```python
from build123d import *

# Parameters (mm, degrees)
ESQUISSE1_W             = 330
ESQUISSE1_H             = 205
BOSS_EXTRU_1_DEPTH      = 30
CHANFREIN1_SIZE         = 30
CHANFREIN1_SIZE2        = 17.320508076
CONG_1_R                = 50
CONG_3_R                = 10
ESQUISSE2_W             = 310
ESQUISSE2_H             = 185
ENL_V_MAT_EXTRU_1_DEPTH = 1
D_GAGEMENT_M42_D        = 4
D_GAGEMENT_M42_DEPTH    = 10
D_GAGEMENT_M42_TIP      = 1.201721238
D_GAGEMENT_M71_D        = 7
D_GAGEMENT_M71_DEPTH    = 5
D_GAGEMENT_M71_TIP      = 2.103012167
ENL_V_MAT_EXTRU_2_DEPTH = 17.320508


with BuildPart() as part:
    # Esquisse1 → Boss.-Extru.1 (new body)
    with BuildSketch(Plane.XY):
        with Locations((165, 102.5)):
            Rectangle(ESQUISSE1_W, ESQUISSE1_H)
    extrude(amount=BOSS_EXTRU_1_DEPTH)

    # Chanfrein1
    chanfrein1_edges = [part.edges().sort_by_distance(p)[0] for p in [
        (165, 205, 0),
        (330, 102.5, 0),
        (165, 0, 0),
        (0, 102.5, 0),
    ]]
    chanfrein1_side = [part.faces().sort_by_distance(p)[0] for p in [
        (165, 102.5, 0),
    ]]
    chamfer(chanfrein1_edges, length=CHANFREIN1_SIZE, length2=CHANFREIN1_SIZE2, reference=chanfrein1_side[0])

    # Congé1
    cong_1_edges = [part.edges().sort_by_distance(p)[0] for p in [
        (315, 15, 8.660254038),
        (15, 15, 8.660254038),
        (315, 190, 8.660254038),
        (15, 190, 8.660254038),
    ]]
    fillet(cong_1_edges, radius=CONG_1_R)

    # Congé3
    cong_3_edges = [part.edges().sort_by_distance(p)[0] for p in [
        (0, 205, 25.524681254),
        (330, 205, 25.524681254),
        (330, 0, 25.524681254),
        (0, 0, 25.524681254),
    ]]
    fillet(cong_3_edges, radius=CONG_3_R)

    # Esquisse2 → Enlèv. mat.-Extru.1 (cut)
    with BuildSketch(Plane.XY.offset(30)):
        with Locations((165, 102.5)):
            Rectangle(ESQUISSE2_W, ESQUISSE2_H)
    extrude(amount=-ENL_V_MAT_EXTRU_1_DEPTH, mode=Mode.SUBTRACT)

    # Dégagement M42
    with Locations(Plane(origin=(0, 0, 0), x_dir=(-1, 0, 0), z_dir=(0, 0, -1))):
        with Locations((-202.5, 65), (-127.5, 140), (-127.5, 65), (-202.5, 140)):
            Hole(D_GAGEMENT_M42_D / 2, depth=D_GAGEMENT_M42_DEPTH)
            with Locations((0, 0, -(D_GAGEMENT_M42_DEPTH + D_GAGEMENT_M42_TIP / 2))):  # 118° drill point
                Cone(0, D_GAGEMENT_M42_D / 2, D_GAGEMENT_M42_TIP, mode=Mode.SUBTRACT)

    # Dégagement M71
    with Locations(Plane(origin=(0, 0, 0), x_dir=(-1, 0, 0), z_dir=(0, 0, -1))):
        with Locations((-215, 152.5), (-115, 152.5), (-165, 42.313793967)):
            Hole(D_GAGEMENT_M71_D / 2, depth=D_GAGEMENT_M71_DEPTH)
            with Locations((0, 0, -(D_GAGEMENT_M71_DEPTH + D_GAGEMENT_M71_TIP / 2))):  # 118° drill point
                Cone(0, D_GAGEMENT_M71_D / 2, D_GAGEMENT_M71_TIP, mode=Mode.SUBTRACT)

    # Esquisse9 → Enlèv. mat.-Extru.2 (cut)
    with BuildSketch(Plane(origin=(0, 0, 0), x_dir=(-1, 0, 0), z_dir=(0, 0, -1))):
        with BuildLine():
            Line((-330, 180), (-297.928932188, 147.928932188))
            ThreePointArc((-297.928932188, 147.928932188), (-295.761204675, 144.6846987), (-295, 140.857864376))
            Line((-295, 140.857864376), (-295, 64.142135624))
            ThreePointArc((-295, 64.142135624), (-295.761204675, 60.3153013), (-297.928932188, 57.071067812))
            Line((-297.928932188, 57.071067812), (-330, 25))
            Line((-330, 25), (-330, 180))
        make_face()
    extrude(amount=-ENL_V_MAT_EXTRU_2_DEPTH, mode=Mode.SUBTRACT)


solid = part.part
```
Geometry: final body of the model. Coordinates: model frame, mm. A direction names the side the tool comes from. Coordinates: 2 decimals unless noted, no trailing zeros. Order: outer loops, then holes, each group sorted by start corner. A loop starts at its lowest first (then second) coordinate and runs counter-clockwise, first axis right, second up. Notation, with made-up numbers: (-27, 63) - (16, 63) arc R19 cw to (16, 79) - close; hole circle Ø8 at (-6.75, 15). An arc over 180 degrees is marked (long way). Return JSON: item names as keys, results as strings. Group by question number.
1. Cut plane B-B (y = 108.5). Output: boundary loops of the cut face in (x, z), plus the area to 3 significant figures.
2. Set-up query: faces 4 (the face through (295.782, 144.735, 8.539)), 5 (the face through (118.233, 151.159, 2.535)), 6 (the face through (163.04, 190.21, 8.78)). Return all of +Z, -Z, +X, -X, +Y, -Y with unobstructed straight access to the full face (end or side cutting, diameter ignored); none if empty.
3. Cut plane A-A (x = 102). Output: boundary loops of the cut face in (y, z).
4. Material intervals for line 1 along Z through (x, y) = (99.5, 168); line 2 along Y through (x, z) = (202, 3); line 3 along Y through (x, z) = (115, 2), sorted ascending. Write a range as [from, to].
5. Pin query (flat end, axial travel): pin 1 (4 mm diameter, centred on x = 156, z = 3, fed in from +Y); pin 2 (1.5 mm diameter, centred on x = 116, z = 12.5, fed in from +Y); pin 3 (6.5 mm diameter, centred on x = 127.5, y = 140, fed in from +Z). Return the tip coordinate at first contact, or that it passes through.
6. Pull-direction query (X, two-part tool) for faces 1 (the face through (310, 45, 10)), 2 (the face through (163, 104, 29)), 3 (the face through (2.85, 3.01, 24.43)); classes: pulls with the +X half, pulls with the -X half, needs draft (parallel to the pull), parting line crosses it, or undercut.
Resolved:
{
 "1": {"outline": "(0, 17.32) - (30, 0) - (295, 0) - (295, 17.32) - (330, 17.32) - (330, 30) - (320, 30) - (320, 29) - (10, 29) - (10, 30) - (0, 30) - close", "area": "8,720 mm²"},
 "2": {"face 4": "-Z, +X", "face 5": "-Z", "face 6": "-Z, +X, -X, +Y"},
 "3": {"outline": "(0, 17.32) - (30, 0) - (175, 0) - (205, 17.32) - (205, 30) - (195, 30) - (195, 29) - (10, 29) - (10, 30) - (0, 30) - close"},
 "4": {"line 1": "z = [0, 29]", "line 2": "y = [24.8, 63.06], [66.94, 138.06], [141.94, 180.2]", "line 3": "y = [26.54, 149], [156, 178.46]"},
 "5": {"pin 1": "stops at y = 183.66", "pin 2": "stops at y = 197.95", "pin 3": "stops at z = 29"},
 "6": {"face 1": "pulls with the +X half", "face 2": "undercut", "face 3": "pulls with the -X half"}
}
